from build123d import *

# Parameters (mm, degrees)
F0_R     = 1.5875
F0_W     = 21.082
F0_H     = 36.83
F1_DEPTH = 1.5875


with BuildPart() as f1:
    # F0 (on Front) → F1 (new body)
    with BuildSketch(Plane.XZ):
        with BuildLine():
            Line((92.487544, 59.78945), (-68.294456, 59.78945))
            ThreePointArc((-68.294456, 59.78945), (-72.784584, 57.929578), (-74.644456, 53.43945))
            Line((-74.644456, 53.43945), (-74.644456, 3.90945))
            ThreePointArc((-74.644456, 3.90945), (-72.784584, -0.580678), (-68.294456, -2.44055))
            Line((-68.294456, -2.44055), (92.487544, -2.44055))
            ThreePointArc((92.487544, -2.44055), (96.977672, -0.580678), (98.837544, 3.90945))
            Line((98.837544, 3.90945), (98.837544, 53.43945))
            ThreePointArc((98.837544, 53.43945), (96.977672, 57.929578), (92.487544, 59.78945))
        make_face()
        with Locations((-68.294456, 3.90945)):
            Circle(F0_R, mode=Mode.SUBTRACT)
        with Locations((92.487544, 3.90945)):
            Circle(F0_R, mode=Mode.SUBTRACT)
        with Locations((-51.403456, 28.67445)):
            Rectangle(F0_W, F0_H, mode=Mode.SUBTRACT)
        with Locations((-26.003456, 28.67445)):
            Rectangle(F0_W, F0_H, mode=Mode.SUBTRACT)
        with Locations((-0.603456, 28.67445)):
            Rectangle(F0_W, F0_H, mode=Mode.SUBTRACT)
        with Locations((-68.294456, 53.43945)):
            Circle(F0_R, mode=Mode.SUBTRACT)
        with Locations((24.796544, 28.67445)):
            Rectangle(F0_W, F0_H, mode=Mode.SUBTRACT)
        with Locations((50.196544, 28.67445)):
            Rectangle(F0_W, F0_H, mode=Mode.SUBTRACT)
        with Locations((75.596544, 28.67445)):
            Rectangle(F0_W, F0_H, mode=Mode.SUBTRACT)
        with Locations((92.487544, 53.43945)):
            Circle(F0_R, mode=Mode.SUBTRACT)
    extrude(amount=F1_DEPTH)


solid = f1.part
Can you work these out from the model? Positions are in its coordinate system, mm. Coordinates: 2 decimals unless noted, no trailing zeros. Order: outer loops, then holes, each group sorted by start corner. A loop starts at its lowest first (then second) coordinate and runs counter-clockwise, first axis right, second up. Notation, with made-up numbers: M 47.5,3 L 68.5,3 A4 ccw 68.5,7 Z; hole C 45,-11 d4. An arc over 180 degrees is marked long. Answer as CSV lines item,"result".
(1) Suppose I cut it at B-B on x = -9.5. Please give me the cut outline in (y, z), plus the area to 3 significant figures.
Geometry check:
outline,"M -1.59,-2.44 L 0,-2.44 L 0,10.26 L -1.59,10.26 Z; M -1.59,47.09 L 0,47.09 L 0,59.79 L -1.59,59.79 Z"
area,"40.3 mm^2"
(2) Suppose I cut it at C-C on y = -1.3. Count the separate pieces of the cut face and the enclosed holes in it, plus the area to 3 significant figures.
Geometry check:
separate pieces,"1"
enclosed holes,"10"
area,"6,070 mm^2"
(3) I'm going to push a flat-ended pin straight in: pin 1 (3.5 mm diameter, centred on x = 92.49, z = 3.91, fed in from +Y). Where does the tip first touch, or does it pass through?
Geometry check:
pin 1,"y = 0"
(4) Please list where these lines run through material, in increasing order: L1, parallel to Z at x = 8, y = -1; L2, parallel to X at y = -1.35, z = 2.5; L3, parallel to X at y = -0.65, z = 56.5.
Geometry check:
L1,"-2.44 to 10.26, 47.09 to 59.79"
L2,"-74.49 to -69.02, -67.56 to 91.76, 93.22 to 98.68"
L3,"-73.86 to 98.05"
(5) If we mould it in two halves opening along Z, with no side actions, what happens to faces 1 (the cylindrical face through (93.954, -0.783, 3.301)), 2 (the flat face through (11, -1.588, 29)), 3 (the cylindrical face through (96.93, -0.78, -0.63))? For each: released by +Z, released by -Z, zero draft, split by the parting line, or undercut.
Geometry check:
face 1,"undercut"
face 2,"zero draft"
face 3,"released by -Z"
(6) Suppose I cut it at A-A on z = 17.5. Please give me the cut outline in (x, y).
Geometry check:
outline,"M -74.64,-1.59 L -61.94,-1.59 L -61.94,0 L -74.64,0 Z; M -40.86,-1.59 L -36.54,-1.59 L -36.54,0 L -40.86,0 Z; M -15.46,-1.59 L -11.14,-1.59 L -11.14,0 L -15.46,0 Z; M 9.94,-1.59 L 14.26,-1.59 L 14.26,0 L 9.94,0 Z; M 35.34,-1.59 L 39.66,-1.59 L 39.66,0 L 35.34,0 Z; M 60.74,-1.59 L 65.06,-1.59 L 65.06,0 L 60.74,0 Z; M 86.14,-1.59 L 98.84,-1.59 L 98.84,0 L 86.14,0 Z"
